Input: part model. Units: mm. Frame: model coordinates. A direction names the side the tool comes from. Round coordinates to 2 decimals unless told otherwise and drop trailing zeros. Order: outer loops, then holes, each group sorted by start corner. A loop starts at its lowest first (then second) coordinate and runs counter-clockwise, first axis right, second up. Notation, with made-up numbers: (23.5, -3) -> (65.5, -3) arc R22 ccw to (65.5, 31) -> close; hole circle Ø1 at (-20.75, 32). An arc over 180 degrees is marked (long way). Use a Markdown table: item, result.
from build123d import *

# Parameters (mm, degrees)
PAD002_DEPTH = 2
PAD003_DEPTH = 3
CHAMFER_SIZE = 1


with BuildPart() as part:
    # Sketch002 → Pad002 (new body)
    with BuildSketch(Plane.XY):
        with BuildLine():
            Line((17.088408, 39.253582), (-79.015923, 39.253582))
            ThreePointArc((-79.015923, 39.253582), (-81.84435, 38.082009), (-83.015923, 35.253582))
            Line((-83.015923, 35.253582), (-83.015923, -8.745983))
            ThreePointArc((-83.015923, -8.745983), (-81.84435, -11.57441), (-79.015923, -12.745983))
            Line((-79.015923, -12.745983), (-22.915418, -12.745983))
            ThreePointArc((-20.086991, -13.917556), (-21.384684, -13.050465), (-22.915418, -12.745983))
            Line((-20.086991, -13.917556), (-1.9847, -32.019847))
            ThreePointArc((-1.9847, -32.019847), (0.843727, -33.191419), (3.672154, -32.019847))
            Line((3.672154, -32.019847), (24.885358, -10.806643))
            ThreePointArc((24.885358, -10.806643), (26.05693, -7.978216), (24.885358, -5.149789))
            Line((24.885358, -5.149789), (22.259981, -2.524412))
            ThreePointArc((21.088408, 0.304015), (21.39289, -1.226719), (22.259981, -2.524412))
            Line((21.088408, 0.304015), (21.088408, 35.253582))
            ThreePointArc((21.088408, 35.253582), (19.916835, 38.082009), (17.088408, 39.253582))
        make_face()
        with BuildLine():
            Line((14.088408, 34.253582), (-76.015923, 34.253582))
            ThreePointArc((-76.015923, 34.253582), (-77.430137, 33.667796), (-78.015923, 32.253582))
            Line((-78.015923, 32.253582), (-78.015923, -5.745983))
            ThreePointArc((-78.015923, -5.745983), (-77.430137, -7.160197), (-76.015923, -7.745983))
            Line((-76.015923, -7.745983), (-20.015923, -7.745983))
            ThreePointArc((-18.601709, -8.331769), (-19.250556, -7.898224), (-20.015923, -7.745983))
            Line((-18.601709, -8.331769), (-0.570487, -26.362992))
            ThreePointArc((-0.570487, -26.362992), (0.843727, -26.948779), (2.257941, -26.362992))
            Line((2.257941, -26.362992), (19.228503, -9.39243))
            ThreePointArc((19.228503, -9.39243), (19.81429, -7.978216), (19.228503, -6.564002))
            Line((19.228503, -6.564002), (16.674194, -4.009694))
            ThreePointArc((16.088408, -2.59548), (16.240649, -3.360847), (16.674194, -4.009694))
            Line((16.088408, -2.59548), (16.088408, 32.253582))
            ThreePointArc((16.088408, 32.253582), (15.502622, 33.667796), (14.088408, 34.253582))
        make_face(mode=Mode.SUBTRACT)
    extrude(amount=-PAD002_DEPTH)

    # Sketch003 (on Face30 of Pad002) → Pad003 (join)
    with BuildSketch(Plane(origin=(0, 0, -2), x_dir=(1, 0, 0), z_dir=(0, 0, -1))):
        with BuildLine():
            Line((-79.015923, 12.745983), (-22.915418, 12.745983))
            ThreePointArc((-22.915418, 12.745983), (-21.384684, 13.050465), (-20.086991, 13.917556))
            Line((-20.086991, 13.917556), (-1.9847, 32.019847))
            ThreePointArc((3.672154, 32.019847), (0.843727, 33.191419), (-1.9847, 32.019847))
            Line((3.672154, 32.019847), (24.885358, 10.806643))
            ThreePointArc((24.885358, 5.149789), (26.05693, 7.978216), (24.885358, 10.806643))
            Line((24.885358, 5.149789), (22.259981, 2.524412))
            ThreePointArc((22.259981, 2.524412), (21.39289, 1.226719), (21.088408, -0.304015))
            Line((21.088408, -0.304015), (21.088408, -35.253582))
            ThreePointArc((17.088408, -39.253582), (19.916835, -38.082009), (21.088408, -35.253582))
            Line((17.088408, -39.253582), (-79.015923, -39.253582))
            ThreePointArc((-83.015923, -35.253582), (-81.84435, -38.082009), (-79.015923, -39.253582))
            Line((-83.015923, -35.253582), (-83.015923, 8.745983))
            ThreePointArc((-79.015923, 12.745983), (-81.84435, 11.57441), (-83.015923, 8.745983))
        make_face()
    extrude(amount=PAD003_DEPTH)

    # Chamfer
    chamfer_edges = [part.edges().sort_by_distance(p)[0] for p in [
        (-83.015923, 13.2538, -5),
        (-81.84435, -11.57441, -5),
        (-50.96567, -12.745983, -5),
        (-21.384684, -13.050465, -5),
        (-11.035845, -22.968701, -5),
        (0.843727, -33.191419, -5),
        (14.278756, -21.413245, -5),
        (26.05693, -7.978216, -5),
        (23.572669, -3.837101, -5),
        (21.39289, -1.226719, -5),
        (21.088408, 17.778798, -5),
        (19.916835, 38.082009, -5),
        (-30.963758, 39.253582, -5),
        (-81.84435, 38.082009, -5),
    ]]
    chamfer(chamfer_edges, length=CHAMFER_SIZE)


with BuildPart() as part_1:
    # Body001 placement: moved
    add(part.part.moved(Location((0, 0, -2.6))))


solid = part_1.part
1) Cut plane B-B on y = 14. Return loops of the section in (x, z), and give its area (3 significant figures).
Results found:
| item | result |
|---|---|
| outline | (-83.02, -6.6) -> (-82.02, -7.6) -> (20.09, -7.6) -> (21.09, -6.6) -> (21.09, -2.6) -> (16.09, -2.6) -> (16.09, -4.6) -> (-78.02, -4.6) -> (-78.02, -2.6) -> (-83.02, -2.6) -> close |
| area | 331 mm² |
2) Line query: L1, parallel to X at y = 6.5, z = -4.15; L2, parallel to Y at x = -65, z = -2.95; L3, parallel to Z at x = 12.5, y = 4.5. Output: solid intervals per line, ascending. Write a range as [from, to].
Results found:
| item | result |
|---|---|
| L1 | x = [-83.02, -78.02], [16.09, 21.09] |
| L2 | y = [-12.75, -7.75], [34.25, 39.25] |
| L3 | z = [-7.6, -4.6] |
3) Pin query (flat end, axial travel): pin 1 Ø18.5 at (x, y) = (-7, 1) entering from +Z; pin 2 Ø0.6 at (x, z) = (-30, -4) entering from -Y; pin 3 Ø2 at (y, z) = (24.5, -4.5) entering from +X. Return the tip coordinate at first contact, or that it passes through.
Results found:
| item | result |
|---|---|
| pin 1 | stops at z = -4.6 |
| pin 2 | stops at y = -12.75 |
| pin 3 | stops at x = 21.09 |
4) Pull-direction query (Y, two-part tool) for faces 1 (the flat face through (-78.016, 14, -4)), 2 (the flat face through (-10.8, -22.5, -7.1)), 3 (the flat face through (-30, 39.254, -5)); classes: +Y half, -Y half, draft (parallel to the pull), parting line (faces both ways), or undercut.
Results found:
| item | result |
|---|---|
| face 1 | undercut |
| face 2 | -Y half |
| face 3 | +Y half |
5) Cut plane C-C on x = -60.5. Return loops of the section in (y, z), and give its area (3 significant figures).
Results found:
| item | result |
|---|---|
| outline | (-12.75, -6.6) -> (-11.75, -7.6) -> (38.25, -7.6) -> (39.25, -6.6) -> (39.25, -2.6) -> (34.25, -2.6) -> (34.25, -4.6) -> (-7.75, -4.6) -> (-7.75, -2.6) -> (-12.75, -2.6) -> close |
| area | 175 mm² |
6) Set-up query: faces 4 (the flat face through (-51, -12.746, -5)), 5 (the conical face through (-81.3, 37.59, -7.33)), 6 (the flat face through (-9.712, -17.221, -3.586)), 7 (the flat face through (21.088, 18, -5)). Return all of +Z, -Z, +X, -X, +Y, -Y with unobstructed straight access to the full face (end or side cutting, diameter ignored); none if empty.
Results found:
| item | result |
|---|---|
| face 4 | +Z, -Z, -X, -Y |
| face 5 | -Z, -X, +Y |
| face 6 | +Z |
| face 7 | +Z, -Z, +X, +Y |
7) Cut plane A-A on z = -5.75. Return loops of the section in (x, y).
Results found:
| item | result |
|---|---|
| outline | (-83.02, -8.75) arc R4 ccw to (-79.02, -12.75) -> (-22.92, -12.75) arc R4 cw to (-20.09, -13.92) -> (-1.98, -32.02) arc R4 ccw to (3.67, -32.02) -> (24.89, -10.81) arc R4 ccw to (24.89, -5.15) -> (22.26, -2.52) arc R4 cw to (21.09, 0.3) -> (21.09, 35.25) arc R4 ccw to (17.09, 39.25) -> (-79.02, 39.25) arc R4 ccw to (-83.02, 35.25) -> close |
8) Cut plane D-D on y = -28. Return loops of the section in (x, z).
Results found:
| item | result |
|---|---|
| outline | (-6, -6.6) -> (-4.59, -7.6) -> (6.28, -7.6) -> (7.69, -6.6) -> (7.69, -2.6) -> (-6, -2.6) -> close |
